CAD build for the part. Positions are in the model's coordinates, mm. A direction names the side the tool comes from. Round coordinates to 2 decimals unless told otherwise and drop trailing zeros. Write each loop counter-clockwise with the first axis right and the second up, starting at its lowest first coordinate (ties: lowest second). Pieces come first, ordered by that corner, then holes. Notation, with made-up numbers: (-15.75, 19.5) -> (15.25, 19.5) arc R20 ccw to (15.25, 28.5) -> close; hole circle Ø7 at (36.5, 80). An arc over 180 degrees is marked (long way). Put each result on its own line as item: value. Start each with the question number.
1. Saw through at D-D on z = 4. List the corners of the cut face in (x, y), and give its area (3 significant figures).
2. Saw through at A-A on y = 15.3. List the corners of the cut face in (x, z).
3. Drill centre lines: line 1 (Y direction, x = 6.5, z = 53); line 2 (Z direction, x = 8, y = 29.2); line 3 (Z direction, x = 10.75, y = -4.5). Where is each one in solid material? Low to high. Write a range as from..to.
4. Saw through at C-C on y = -0.5. List the corners of the cut face in (x, z).
5. Pull direction Z, two halves, no side cores. Call faces 1 (the flat face through (8, 0, -39)), 2 (the flat face through (5, 3.8, -3)), 3 (the flat face through (6, -34.2, 25)): pulls with the +Z half, pulls with the -Z half, needs draft (parallel to the pull), parting line crosses it, or undercut.
6. Flat gauge pins, fed straight in: P1, Ø3, axis at y = -29.2, z = -34, coming from the +X side; P2, Ø5, axis at y = 15.3, z = 42.1, coming from the -X side; P3, Ø1, axis at x = 14, z = 27.5, coming from the -Y side. Where does each tip first touch, or does it go through?
7. Saw through at B-B on z = 71.5. List the corners of the cut face in (x, y), and give its area (3 significant figures).
8. 3-axis set-ups, long thin cutter, end or side, ignore diameter. For faces 4 (the cylindrical face through (7.1, -29.38, -32.61)), 5 (the flat face through (6, 3.8, 54)), 6 (the cylindrical face through (15.01, -26.72, -33.22)): which of +Z, -Z, +X, -X, +Y, -Y reach the whole face in a straight line?
from build123d import *

# Parameters (mm, degrees)
SKETCH016_W     = 68.4
SKETCH016_H     = 129
PAD004_DEPTH    = 16
FILLET002_R     = 4
SKETCH017_R     = 1.4
POCKET016_DEPTH = 16
SKETCH018_R     = 2.6
POCKET017_DEPTH = 2
POCKET018_DEPTH = 11
SKETCH020_W     = 21
SKETCH020_H     = 52.4
POCKET019_DEPTH = 3
SKETCH021_W     = 6
SKETCH021_H     = 3
POCKET020_DEPTH = 1
SKETCH022_W     = 2
SKETCH022_H     = 11.5
PAD005_DEPTH    = 1.2
SKETCH023_R     = 2
SKETCH023_R_2   = 1.5
POCKET021_DEPTH = 5


with BuildPart() as part:
    # Sketch016 → Pad004 (new body)
    with BuildSketch(Plane.YZ):
        with Locations((0, 25.5)):
            Rectangle(SKETCH016_W, SKETCH016_H)
    extrude(amount=PAD004_DEPTH)

    # Fillet002
    fillet002_edges = [part.edges().sort_by_distance(p)[0] for p in [
        (16, -34.2, 25.5),
        (16, 34.2, 25.5),
    ]]
    fillet(fillet002_edges, radius=FILLET002_R)

    # Sketch017 (on Face8 of Fillet002) → Pocket016 (cut)
    with BuildSketch(Plane.YZ.offset(16)):
        with Locations((-29.2, 85)):
            Circle(SKETCH017_R)
        with Locations((29.2, 85)):
            Circle(SKETCH017_R)
        with Locations((29.2, -34)):
            Circle(SKETCH017_R)
        with Locations((-29.2, -34)):
            Circle(SKETCH017_R)
    extrude(amount=-POCKET016_DEPTH, mode=Mode.SUBTRACT)

    # Sketch018 (on Face8 of Pocket016) → Pocket017 (cut)
    with BuildSketch(Plane.YZ.offset(16)):
        with Locations((-29.2, 85)):
            Circle(SKETCH018_R)
        with Locations((29.2, 85)):
            Circle(SKETCH018_R)
        with Locations((29.2, -34)):
            Circle(SKETCH018_R)
        with Locations((-29.2, -34)):
            Circle(SKETCH018_R)
    extrude(amount=-POCKET017_DEPTH, mode=Mode.SUBTRACT)

    # Sketch019 (on Face4 of Pocket017) → Pocket018 (cut)
    with BuildSketch(Plane(origin=(0, 0, 0), x_dir=(0, 1, 0), z_dir=(-1, 0, 0))):
        with BuildLine():
            ThreePointArc((25.8, 34), (26.795837, 31.595837), (29.2, 30.6))
            Line((32.2, 30.6), (29.2, 30.6))
            Line((32.2, -82.6), (32.2, 30.6))
            Line((29.2, -82.6), (32.2, -82.6))
            ThreePointArc((29.2, -82.6), (27.502944, -83.302944), (26.8, -85))
            Line((26.8, -89), (26.8, -85))
            Line((-25.8, -89), (26.8, -89))
            Line((-25.8, -89), (-25.8, -85))
            ThreePointArc((-25.8, -85), (-26.795837, -82.595837), (-29.2, -81.6))
            Line((-32.2, -81.6), (-29.2, -81.6))
            Line((-32.2, -77.5), (-32.2, -81.6))
            Line((3.8, -77.5), (-32.2, -77.5))
            Line((3.8, -30.5), (3.8, -77.5))
            Line((1.8, -30.5), (3.8, -30.5))
            Line((1.8, -75.5), (1.8, -30.5))
            Line((-32.2, -75.5), (1.8, -75.5))
            Line((-32.2, 24.5), (-32.2, -75.5))
            Line((1.8, 24.5), (-32.2, 24.5))
            Line((1.8, 24.5), (1.8, -20.5))
            Line((1.8, -20.5), (3.8, -20.5))
            Line((3.8, 26.5), (3.8, -20.5))
            Line((-32.2, 26.5), (3.8, 26.5))
            Line((-32.2, 30.6), (-32.2, 26.5))
            Line((-29.2, 30.6), (-32.2, 30.6))
            ThreePointArc((-29.2, 30.6), (-26.795837, 31.595837), (-25.8, 34))
            Line((-25.8, 34), (-25.8, 37))
            Line((-25.8, 37), (25.8, 37))
            Line((25.8, 37), (25.8, 34))
        make_face()
    extrude(amount=-POCKET018_DEPTH, mode=Mode.SUBTRACT)

    # Sketch020 (on Face49 of Pocket018) → Pocket019 (cut)
    with BuildSketch(Plane(origin=(11, 0, 0), x_dir=(0, 1, 0), z_dir=(-1, 0, 0))):
        with Locations((15.3, -62.8)):
            Rectangle(SKETCH020_W, SKETCH020_H)
    extrude(amount=-POCKET019_DEPTH, mode=Mode.SUBTRACT)

    # Sketch021 (on Face50 of Pocket019) → Pocket020 (cut)
    with BuildSketch(Plane.YX.offset(-89)):
        with BuildLine():
            ThreePointArc((12.3, 14), (10.8, 12.5), (12.3, 11))
            Line((12.3, 11), (18.3, 11))
            ThreePointArc((18.3, 11), (19.8, 12.5), (18.3, 14))
            Line((12.3, 14), (18.3, 14))
        make_face()
        with Locations((15.3, 7.5)):
            Rectangle(SKETCH021_W, SKETCH021_H)
    extrude(amount=-POCKET020_DEPTH, mode=Mode.SUBTRACT)

    # Sketch022 (on Face60 of Pocket020) → Pad005 (join)
    with BuildSketch(Plane(origin=(11, 0, 0), x_dir=(0, 1, 0), z_dir=(-1, 0, 0))):
        with Locations((2.8, -83.25)):
            Rectangle(SKETCH022_W, SKETCH022_H)
        Polygon((1.8, -33.6), (28.8, -33.6), (28.8, -77.5), (26.8, -77.5), (26.8, -35.6), (1.8, -35.6), align=None)
    extrude(amount=PAD005_DEPTH)

    # Sketch023 (on Face55 of Pad005) → Pocket021 (cut)
    with BuildSketch(Plane(origin=(14, 0, 0), x_dir=(0, 1, 0), z_dir=(-1, 0, 0))):
        with Locations((15.3, -42.1)):
            Circle(SKETCH023_R)
        with Locations((10.3, -42.1)):
            Circle(SKETCH023_R_2)
        with Locations((20.3, -42.1)):
            Circle(SKETCH023_R_2)
        with Locations((11.3, -68.5)):
            Circle(SKETCH023_R_2)
    extrude(amount=-POCKET021_DEPTH, mode=Mode.SUBTRACT)


solid = part.part
Return value:
1. outline: (0, -34.2) -> (12, -34.2) arc R4 ccw to (16, -30.2) -> (16, 30.2) arc R4 ccw to (12, 34.2) -> (0, 34.2) -> (0, 32.2) -> (11, 32.2) -> (11, 3.8) -> (0, 3.8) -> (0, 1.8) -> (11, 1.8) -> (11, -32.2) -> (0, -32.2) -> close
1. area: 401 mm^2
2. outline: (0, -39) -> (16, -39) -> (16, 40.1) -> (14, 40.1) -> (14, 36.6) -> (11, 36.6) -> (11, 35.6) -> (9.8, 35.6) -> (9.8, 33.6) -> (11, 33.6) -> (11, -37) -> (0, -37) -> close; (0, 89) -> (6, 89) -> (6, 90) -> (0, 90) -> close; (9, 89) -> (11, 89) -> (11, 90) -> (9, 90) -> close; (14, 44.1) -> (16, 44.1) -> (16, 90) -> (14, 90) -> close
3. line 1: y = -34.2..-32.2, 1.8..3.8, 32.2..34.2
3. line 2: z = -39..-35.4, -32.6..-30.6, 82.6..83.6, 86.4..90
3. line 3: z = -39..-37, -26.5..-24.5, 75.5..77.5, 89..90
4. outline: (0, -39) -> (16, -39) -> (16, 90) -> (0, 90) -> (0, 89) -> (11, 89) -> (11, 77.5) -> (0, 77.5) -> (0, 75.5) -> (11, 75.5) -> (11, -24.5) -> (0, -24.5) -> (0, -26.5) -> (11, -26.5) -> (11, -37) -> (0, -37) -> close
5. face 1: pulls with the -Z half
5. face 2: undercut
5. face 3: needs draft
6. P1: stops at x = 14
6. P2: stops at x = 14
6. P3: stops at y = -33.91
7. outline: (0, -34.2) -> (12, -34.2) arc R4 ccw to (16, -30.2) -> (16, 30.2) arc R4 ccw to (12, 34.2) -> (0, 34.2) -> (0, 32.2) -> (11, 32.2) -> (11, 28.8) -> (9.8, 28.8) -> (9.8, 26.8) -> (11, 26.8) -> (11, 25.8) -> (14, 25.8) -> (14, 4.8) -> (11, 4.8) -> (11, 3.8) -> (0, 3.8) -> (0, 1.8) -> (11, 1.8) -> (11, -32.2) -> (0, -32.2) -> close
7. area: 341 mm^2
8. face 4: +X, -X
8. face 5: -X
8. face 6: +X
